Autodesk Inventor part; units mm, degrees
ref_plane "Work Plane1" through (-12.5, 0, 0) normal (-1, 0, 0) x (0, 0, 1)
ref_plane "YZ Plane" through (0, 0, 0) normal (1, 0, 0) x (0, 1, 0)
ref_plane "XZ Plane" through (0, 0, 0) normal (0, 1, 0) x (-1, 0, 0)
sketch "Sketch5" plane through (0, 0, 0) normal (0, 0, 1) x (1, 0, 0)
  line L0 (71.5, 5) -> (71.5, 11.15)
  line L1 (71.5, 11.15) -> (77.5, 11.15)
  line L2 (77.5, 11.15) -> (77.5, 14.5)
  line L3 (77.5, 14.5) -> (67.5, 14.5)
  line L4 (67.5, 14.5) -> (67.5, 14.2)
  line L5 (66, 12.7) -> (-12.5, 12.7)
  line L6 (71.5, 5) -> (-12.5, 5)
  line L7 (-12.5, 5) -> (-12.5, 12.7)
  line L8 (0, 0) -> (106.4906, 0) construction
  line L9 (67.5, 14.2) -> (67.5, 14.2)
  arc A0 (66, 12.7) -> (67.5, 14.2) centre (66, 14.2) ccw
  line L10 (35.25, 16.2) -> (60.7131, 16.2)
  point P0 (67.5, 12.7)
  point P1 (67.5, 14.5)
  point P2 (67.5, 14.2)
  dimension "d12" = 5
  dimension "d14" = 6
  dimension "d16" = 11.15
  dimension "d17" = 14.5
  dimension "d19" = 10
  dimension "d27" = 80
  dimension "d28" = 1.5
  dimension "d29" = 12.7
  dimension "d30" = 3.5
revolve "Revolution1" add sketch "Sketch5" angle 360 about axis through (0, 0, 0) along (1, 0, 0)
ref_plane "Work Plane1" through (-12.5, 0, 0) normal (-1, 0, 0) x (0, 0, 1)
mirror "Mirror1" about plane through (-12.5, 0, 0) normal (-1, 0, 0) of "Revolution1"
properties part number "12111_Proximal Roller_V1" material "ABS Plastic"
Check sheet for the modelled part. Datum: model origin and axes. Units: mm. A direction names the side the tool comes from. Coordinates: 2 decimals unless noted, no trailing zeros. Loops run counter-clockwise (first coordinate to the right, second up) from the corner with the lowest first, then second, coordinate; pieces in that order, holes last. Notation, with made-up numbers: (59, 46.25) -> (86, 46.25) arc R24 ccw to (86, 83.25) -> close; hole circle Ø11 at (1, 38). An arc over 180 degrees is marked (long way). Write item = value, one per line. Start each with the question number.
1. Section check A-A on z = 0. Record the cut outline in (x, y).
2. Section check C-C on x = -37. Record the cut outline in (y, z).
3. Tool access check on faces 1 (the flat face through (77.5, -3, -11)), 2 (the flat face through (71.5, 2, -5)), 3 (the cylindrical face through (-99.542, 10.635, -3.349)). Record the directions out of +Z, -Z, +X, -X, +Y, -Y that give a thin tool (end or side, any length) a straight path to the whole face; none if there is none.
4. Draft check along X on faces 4 (the cylindrical face through (-11.4, -2.75, -12.4)), 5 (the flat face through (-96.5, -2, -5)), 6 (the cylindrical face through (74.542, 10.635, 3.349)). Enter one of: released by +X, released by -X, zero draft, split by the parting line, or undercut.
5. Material ranges on line 1 (Z direction, x = -101.1, y = 0); line 2 (Z direction, x = -42, y = 0); line 3 (X direction, y = 1.25, z = -8), recorded low to high.
6. Depth check by flat-ended pin: P1, Ø10, axis at x = -10.5, z = 9, coming from the -Y side; P2, Ø6, axis at y = 1, z = 2, coming from the -X side; P3, Ø11, axis at y = -3, z = -5, coming from the +X side; P4, Ø8, axis at x = -9.5, y = -10, coming from the +Z side. Enter the tip coordinate at first touch or a pass-through.
Responses:
q1.outline = (-102.5, -14.5) -> (-92.5, -14.5) -> (-92.5, -14.2) arc R1.5 cw to (-91, -12.7) -> (66, -12.7) arc R1.5 cw to (67.5, -14.2) -> (67.5, -14.5) -> (77.5, -14.5) -> (77.5, -11.15) -> (71.5, -11.15) -> (71.5, -5) -> (-96.5, -5) -> (-96.5, -11.15) -> (-102.5, -11.15) -> close; (-102.5, 11.15) -> (-96.5, 11.15) -> (-96.5, 5) -> (71.5, 5) -> (71.5, 11.15) -> (77.5, 11.15) -> (77.5, 14.5) -> (67.5, 14.5) -> (67.5, 14.2) arc R1.5 cw to (66, 12.7) -> (-91, 12.7) arc R1.5 cw to (-92.5, 14.2) -> (-92.5, 14.5) -> (-102.5, 14.5) -> close
q2.outline = circle Ø25.4 at (0, 0); hole circle Ø10 at (0, 0)
q3.face_1 = +Z, -Z, +X, +Y, -Y
q3.face_2 = +X
q3.face_3 = -X
q4.face_4 = undercut
q4.face_5 = released by -X
q4.face_6 = zero draft
q5.line_1 = -14.5 to -11.15, 11.15 to 14.5
q5.line_2 = -12.7 to -5, 5 to 12.7
q5.line_3 = -96.5 to 71.5
q6.P1 = -12.05
q6.P2 = -96.5
q6.P3 = 77.5
q6.P4 = 11.19
